Can you work these out from the model? Positions are in its coordinate system, mm. A direction names the side the tool comes from. Round coordinates to 2 decimals unless told otherwise and drop trailing zeros. Loops run counter-clockwise (first coordinate to the right, second up) from the corner with the lowest first, then second, coordinate; pieces in that order, holes last.
from build123d import *

# Parameters (mm, degrees)
SKETCH1_W                = 21
SKETCH1_H                = 49.25
BOSS_EXTRUDE1_DEPTH      = 20
SKETCH4_R                = 7.5
BOSS_EXTRUDE2_DEPTH      = 6
BOSS_EXTRUDE2_DEPTH_BACK = 63.25
SKETCH2_W                = 50
SKETCH2_H                = 112.412407925
SKETCH2_R                = 12.5
CUT_EXTRUDE1_DEPTH       = 110.803517703
CUT_EXTRUDE1_DEPTH_BACK  = 110.803517703
SKETCH5_W                = 20
SKETCH5_H                = 49.25
CUT_EXTRUDE2_DEPTH       = 103.250382029
CUT_EXTRUDE3_DEPTH       = 110.803517703
SKETCH7_W                = 9.75
SKETCH7_H                = 14.35
BOSS_EXTRUDE3_DEPTH      = 22
CUT_EXTRUDE4_REACH       = 99.528
SKETCH8_R                = 1.25
SKETCH9_R                = 2.25
CUT_EXTRUDE5_DEPTH       = 26.4
SKETCH10_R               = 0.6
SKETCH10_R_2             = 0.95
CUT_EXTRUDE6_DEPTH       = 2
SKETCH17_R               = 3.5
SKETCH17_R_2             = 0.95
CUT_EXTRUDE11_DEPTH      = 1
SKETCH11_R               = 1
CUT_EXTRUDE7_DEPTH       = 2
CUT_EXTRUDE8_DEPTH       = 4
CUT_EXTRUDE9_DEPTH       = 82.485524021
SKETCH14_R               = 12.5
SKETCH14_R_2             = 6.5
BOSS_EXTRUDE4_DEPTH      = 4
SKETCH16_R               = 3
CUT_EXTRUDE10_DEPTH      = 4
SKETCH18_R               = 11
BOSS_EXTRUDE5_DEPTH      = 1.9
SKETCH19_R               = 11
BOSS_EXTRUDE6_DEPTH      = 1.9
SKETCH20_R               = 4
CUT_EXTRUDE12_DEPTH      = 75
SKETCH22_R               = 45
CUT_EXTRUDE14_DEPTH      = 8


with BuildPart() as part:
    # Sketch1 → Boss-Extrude1 (new, symmetric)
    with BuildSketch(Plane.YZ):
        Polygon((-12.5, 24.625), (-12.5, 28.625), (87.5, 28.625), (87.5, 24.625), (58.5, 24.625), (58.5, -24.625), (87.5, -24.625), (87.5, -28.625), (-12.5, -28.625), (-12.5, -24.625), (22.5, -24.625), (22.5, 24.625), align=None)
        with Locations((41, 0)):
            Rectangle(SKETCH1_W, SKETCH1_H, mode=Mode.SUBTRACT)
    extrude(amount=BOSS_EXTRUDE1_DEPTH, both=True)

    # Sketch4 → Boss-Extrude2 (add, two sides)
    with BuildSketch(Plane(origin=(0, 0, -28.625), x_dir=(1, 0, 0), z_dir=(0, 0, -1))) as boss_extrude2_sk:
        with Locations(Location((0, 0, 0), (0, 0, 180))):
            Circle(SKETCH4_R)
    extrude(amount=BOSS_EXTRUDE2_DEPTH)
    extrude(boss_extrude2_sk.sketch, amount=-BOSS_EXTRUDE2_DEPTH_BACK)

    # Sketch2 → Cut-Extrude1 (cut, two sides)
    with BuildSketch(Plane(origin=(0, 0, -28.625), x_dir=(1, 0, 0), z_dir=(0, 0, -1))) as cut_extrude1_sk:
        with Locations((0, -36.293796038)):
            Rectangle(SKETCH2_W, SKETCH2_H)
        with BuildLine():
            Line((20, -0.087592075), (20, -72.5))
            ThreePointArc((20, -72.5), (0, -87.5), (-20, -72.5))
            Line((-20, -72.5), (-20, -0.087592075))
            ThreePointArc((-20, -0.087592075), (0, 12.5), (20, -0.087592075))
        make_face(mode=Mode.SUBTRACT)
        with Locations(Location((0, -72.5, 0), (0, 0, 270))):
            Circle(SKETCH2_R)
    extrude(amount=CUT_EXTRUDE1_DEPTH, mode=Mode.SUBTRACT)
    extrude(cut_extrude1_sk.sketch, amount=-CUT_EXTRUDE1_DEPTH_BACK, mode=Mode.SUBTRACT)

    # Sketch5 → Cut-Extrude2 (cut, through all)
    with BuildSketch(Plane.YZ.offset(20)):
        Rectangle(SKETCH5_W, SKETCH5_H)
    extrude(amount=-CUT_EXTRUDE2_DEPTH, mode=Mode.SUBTRACT)

    # Sketch6 → Cut-Extrude3 (cut, through all)
    with BuildSketch(Plane(origin=(0, 0, -28.625), x_dir=(1, 0, 0), z_dir=(0, 0, -1))):
        with BuildLine():
            Line((-12, 5.343628911), (-12, -13.048253679))
            ThreePointArc((-12, -13.048253679), (-13.67544468, -17.947233164), (-18, -20.794220371))
            ThreePointArc((-18, -20.794220371), (-19.196771953, -21.416398141), (-20, -22.5))
            Line((-20, -22.5), (-20, 15.418169496))
            Line((-20, 15.418169496), (0, 15.418169496))
            Line((0, 15.418169496), (0, 12.5))
            ThreePointArc((0, 12.5), (-4.185625792, 12.101526483), (-8.220875011, 10.92042185))
            ThreePointArc((-8.220875011, 10.92042185), (-10.966225922, 8.711952128), (-12, 5.343628911))
        make_face()
    extrude(amount=-CUT_EXTRUDE3_DEPTH, mode=Mode.SUBTRACT)

    # Sketch7 → Boss-Extrude3 (add)
    with BuildSketch(Plane(origin=(0, 58.5, 0), x_dir=(-1, 0, 0), z_dir=(0, 1, 0))):
        with Locations((15.125, 3.65)):
            Rectangle(SKETCH7_W, SKETCH7_H)
    extrude(amount=BOSS_EXTRUDE3_DEPTH)

    # Sketch8 → Cut-Extrude4 (cut, up to next)
    with BuildSketch(Plane(origin=(0, 0, -3.525), x_dir=(1, 0, 0), z_dir=(0, 0, -1)), mode=Mode.PRIVATE) as cut_extrude4_sk1:
        with Locations(Location((-14, -67.5, 0), (0, 0, 270))):
            Circle(SKETCH8_R)
    cut_extrude4_tool1 = extrude(cut_extrude4_sk1.sketch, amount=-CUT_EXTRUDE4_REACH, mode=Mode.PRIVATE) & part.part
    # Sketch8 → Cut-Extrude4 (cut, up to next)
    with BuildSketch(Plane(origin=(0, 0, -3.525), x_dir=(1, 0, 0), z_dir=(0, 0, -1)), mode=Mode.PRIVATE) as cut_extrude4_sk2:
        with Locations(Location((-14, -77.5, 0), (0, 0, 270))):
            Circle(SKETCH8_R)
    cut_extrude4_tool2 = extrude(cut_extrude4_sk2.sketch, amount=-CUT_EXTRUDE4_REACH, mode=Mode.PRIVATE) & part.part
    add(cut_extrude4_tool1.solids().sort_by_distance((-14, 67.5, -3.525))[0], mode=Mode.SUBTRACT)
    add(cut_extrude4_tool2.solids().sort_by_distance((-14, 77.5, -3.525))[0], mode=Mode.SUBTRACT)

    # Sketch9 → Cut-Extrude5 (cut)
    with BuildSketch(Plane(origin=(0, 0, -28.625), x_dir=(1, 0, 0), z_dir=(0, 0, -1))):
        with Locations(Location((-14, -77.5, 0), (0, 0, 180))):
            Circle(SKETCH9_R)
        with Locations(Location((-14, -67.5, 0), (0, 0, 90))):
            Circle(SKETCH9_R)
    extrude(amount=-CUT_EXTRUDE5_DEPTH, mode=Mode.SUBTRACT)

    # Sketch10 → Cut-Extrude6 (cut)
    with BuildSketch(Plane.XY.offset(-24.625)):
        with BuildLine():
            Line((-0.917974412, 6.434852211), (15.551094055, 8.784274226))
            ThreePointArc((15.551094055, 8.784274226), (18.793852416, 6.840402867), (17.559251818, 3.266906118))
            Line((17.559251818, 3.266906118), (3.433034074, -5.519445357))
            ThreePointArc((3.433034074, -5.519445357), (2.223130932, -6.108002035), (0.917974412, -6.434852211))
            Line((0.917974412, -6.434852211), (-15.551094055, -8.784274226))
            ThreePointArc((-15.551094055, -8.784274226), (-18.793852416, -6.840402867), (-17.559251818, -3.266906118))
            Line((-17.559251818, -3.266906118), (-3.433034074, 5.519445357))
            ThreePointArc((-3.433034074, 5.519445357), (-2.223130932, 6.108002035), (-0.917974412, 6.434852211))
        make_face()
        with Locations((12.309973332, 4.480463878)):
            Circle(SKETCH10_R, mode=Mode.SUBTRACT)
        with Locations((9.584864732, 3.488605462)):
            Circle(SKETCH10_R, mode=Mode.SUBTRACT)
        with Locations((6.859756132, 2.496747046)):
            Circle(SKETCH10_R, mode=Mode.SUBTRACT)
        Circle(SKETCH10_R_2, mode=Mode.SUBTRACT)
    extrude(amount=-CUT_EXTRUDE6_DEPTH, mode=Mode.SUBTRACT)

    # Sketch17 → Cut-Extrude11 (cut)
    with BuildSketch(Plane.XY.offset(-26.625)):
        Circle(SKETCH17_R)
        Circle(SKETCH17_R_2, mode=Mode.SUBTRACT)
    extrude(amount=-CUT_EXTRUDE11_DEPTH, mode=Mode.SUBTRACT)

    # Sketch11 → Cut-Extrude7 (cut)
    with BuildSketch(Plane.XY.offset(-26.625)):
        with Locations((14.659204884, 5.335514236)):
            Circle(SKETCH11_R)
        with Locations(Location((-6.859756132, -2.496747046, 0), (0, 0, 282.284944741))):
            Circle(SKETCH11_R)
    extrude(amount=-CUT_EXTRUDE7_DEPTH, mode=Mode.SUBTRACT)

    # Sketch12 → Cut-Extrude8 (cut)
    with BuildSketch(Plane.XY.offset(28.625)):
        with BuildLine():
            Line((0, -12.5), (0, -18.039119765))
            Line((0, -18.039119765), (20, -18.039119765))
            Line((20, -18.039119765), (20, 21.429096263))
            ThreePointArc((20, 21.429096263), (19.196193013, 20.360986537), (18.008206922, 19.748081074))
            ThreePointArc((18.008206922, 19.748081074), (13.678040469, 16.902328803), (12, 12))
            Line((12, 12), (12, -3.925954614))
            ThreePointArc((12, -3.925954614), (10.465352752, -8.637558778), (6.450196551, -11.541500351))
            ThreePointArc((6.450196551, -11.541500351), (3.264426341, -12.285407289), (0, -12.5))
        make_face()
    extrude(amount=-CUT_EXTRUDE8_DEPTH, mode=Mode.SUBTRACT)

    # Sketch13 → Cut-Extrude9 (cut, through all)
    with BuildSketch(Plane(origin=(0, 58.5, 0), x_dir=(-1, 0, 0), z_dir=(0, 1, 0))):
        with BuildLine():
            Line((-20, 24.625), (-20, -24.625))
            ThreePointArc((-20, -24.625), (-12.664431165, 0), (-20, 24.625))
        make_face()
    extrude(amount=-CUT_EXTRUDE9_DEPTH, mode=Mode.SUBTRACT)

    # Sketch14 → Boss-Extrude4 (add)
    with BuildSketch(Plane.XY.offset(28.625)):
        with Locations(Location((0, 72.5, 0), (0, 0, 180))):
            Circle(SKETCH14_R)
        with Locations((0, 72.5)):
            Circle(SKETCH14_R_2, mode=Mode.SUBTRACT)
    extrude(amount=-BOSS_EXTRUDE4_DEPTH)

    # Sketch16 → Cut-Extrude10 (cut)
    with BuildSketch(Plane.XY.offset(28.625)):
        with Locations((0, 79.8)):
            Circle(SKETCH16_R)
    extrude(amount=-CUT_EXTRUDE10_DEPTH, mode=Mode.SUBTRACT)

    # Sketch18 → Boss-Extrude5 (add)
    with BuildSketch(Plane.XY.offset(34.625)):
        Circle(SKETCH18_R)
    extrude(amount=-BOSS_EXTRUDE5_DEPTH)

    # Sketch19 → Boss-Extrude6 (add)
    with BuildSketch(Plane(origin=(0, 0, -34.625), x_dir=(1, 0, 0), z_dir=(0, 0, -1))):
        Circle(SKETCH19_R)
    extrude(amount=-BOSS_EXTRUDE6_DEPTH)

    # Sketch20 → Cut-Extrude12 (cut)
    with BuildSketch(Plane.XZ.offset(-22.5)):
        with Locations(Location((0, 0, 0), (0, 0, 270))):
            Circle(SKETCH20_R)
    extrude(amount=-CUT_EXTRUDE12_DEPTH, mode=Mode.SUBTRACT)

    # Sketch22 → Cut-Extrude14 (cut)
    with BuildSketch(Plane.XZ.offset(-22.5)):
        with Locations((-57.664431165, 0)):
            Circle(SKETCH22_R)
    extrude(amount=-CUT_EXTRUDE14_DEPTH, mode=Mode.SUBTRACT)


solid = part.part
(1) If we section it at B-B, the plane y = 39: List the corners of the cut face in (x, z) for me (3 decimals).
Worked answers:
outline: (-20, -28.625) - (20, -28.625) - (20, -24.625) - (-20, -24.625) - close; (-20, 24.625) - (20, 24.625) - (20, 28.625) - (-20, 28.625) - close
(2) For faces 1 (the cylindrical face through (-2.24, 6.1, -25.61)), 2 (the flat face through (12, 4, 27)), 3 (the cylindrical face through (-13.512, 75.304, -2.884)), which set-ups out of +Z, -Z, +X, -X, +Y, -Y let a thin tool reach every point of the face, with its end or its side?
Worked answers:
face 1: none
face 2: +Z, +X, -Y
face 3: -Z
(3) If I drill on line 1 (Z direction, x = -14.5, y = 51) (3 decimals); line 2 (Y direction, x = 11, z = -16.5); line 3 (X direction, y = 77.5, z = 1.5), over which ranges is the centre line in solid material (lowest first)?
Worked answers:
line 1: z = -28.625 to -24.625, 24.625 to 28.625
line 2: y = 22.5 to 30.5, 51.5 to 58.5
line 3: x = -20 to -15.25, -12.75 to -10.25
(4) If we section it at C-C, the plane y = 67.5: State how many separate pieces and enclosed holes the cut face has, then the cut area to 3 significant figures.
Worked answers:
separate pieces: 7
enclosed holes: 0
area: 279 mm2
(5) Will these pins go through, and if not, where does the flat tip stop? P1, Ø14.5, axis at x = 6, y = 69.5, coming from the -Z side (3 decimals); P2, Ø2, axis at y = -0.5, z = 26.5, coming from the -X side; P3, Ø1, axis at x = -13, y = 61.5, coming from the +Z side (3 decimals).
Worked answers:
P1: stops at z = -28.625
P2: stops at x = -12
P3: stops at z = 28.625
(6) If we section it at D-D, the plane z = 22: List the corners of the cut face in (x, y) for me, then the cut area to 3 significant figures.
Worked answers:
outline: (-20, 51.5) - (18.41, 51.5) - (18.41, 58.5) - (-20, 58.5) - close; (-18.41, 22.5) - (18.41, 22.5) - (18.41, 30.5) - (-18.41, 30.5) - close
area: 563 mm2
(7) If we mould it in two halves opening along X, with no side actions, what happens to faces 4 (the cylindrical face through (-14.099, 69.748, -26.653)), 5 (the flat face through (5, 9, -24.625)), 6 (the cylindrical face through (-13.62, 68.69, 4.21)), 7 (the flat face through (-12, 4, 27))? For each: released by +X, released by -X, zero draft, split by the parting line, or undercut.
Worked answers:
face 4: undercut
face 5: zero draft
face 6: undercut
face 7: released by -X
(8) If we section it at A-A, the plane z = 0: List the corners of the cut face in (x, y) for me, then the cut area to 3 significant figures.
Worked answers:
outline: (-20, 51.5) - (-4, 51.5) - (-4, 58.5) - (-10.25, 58.5) - (-10.25, 80.5) - (-20, 80.5) - close; (-12.66, 22.5) - (-4, 22.5) - (-4, 30.5) - (-12.66, 30.5) - close; (4, 22.5) - (12.66, 22.5) - (12.66, 30.5) - (4, 30.5) - close; (4, 51.5) - (12.66, 51.5) - (12.66, 58.5) - (4, 58.5) - close; hole circle Ø2.5 at (-14, 67.5); hole circle Ø2.5 at (-14, 77.5)
area: 516 mm2
